```python
from build123d import *

# Parameters (mm, degrees)
BOSS_EXTRUDE1_DEPTH = 5


with BuildPart() as part:
    # Sketch1 → Boss-Extrude1 (new body)
    with BuildSketch(Plane(origin=(0, 0, 0), x_dir=(1, 0, 0), z_dir=(0, 1, 0))):
        with BuildLine():
            ThreePointArc((-40.530858986, 10), (-2.570543478, 38.792166423), (35.38977203, 10))
            Line((35.38977203, 10), (21.844456522, 10))
            Line((21.844456522, 10), (21.844456522, 0))
            Line((21.844456522, 0), (-26.985543478, 0))
            Line((-26.985543478, 0), (-26.985543478, 10))
            Line((-26.985543478, 10), (-40.530858986, 10))
        make_face()
    extrude(amount=BOSS_EXTRUDE1_DEPTH)


solid = part.part
```
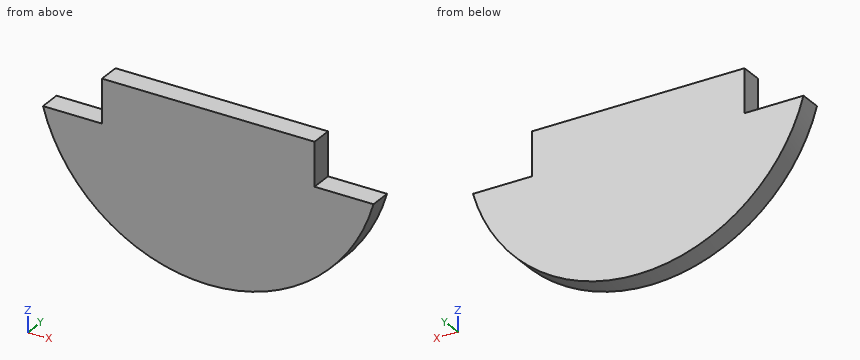
Check sheet for the modelled part. Datum: model origin and axes. Units: mm. Give positions to 0.01 mm unless a question says otherwise; leave off trailing zeros. Loops run counter-clockwise (first coordinate to the right, second up) from the corner with the lowest first, then second, coordinate; pieces in that order, holes last. Notation, with made-up numbers: (-21.5, -37) - (4.5, -37) arc R17 ccw to (4.5, -29) - close; hole circle Ø1 at (43.5, 44.5). An arc over 180 degrees is marked (long way). One line per question, with ' | ' between items. Start each with the question number.
1. Cross-section at C-C, the plane x = 26. Enter the section's corners in (y, z).
2. Gauge pin test, flat ends, axial feed: pin 1 Ø2 at (y, z) = (4.5, -26.5) entering from -X; pin 2 Ø1.5 at (y, z) = (1.5, -6) entering from -X. Record the tip position at first contact, or that the pin passes through.
3. Cross-section at B-B, the plane z = -5.5. Enter the section's corners in (x, y), plus the area to 3 significant figures.
4. Material ranges on line 1 along X through (y, z) = (2.1, -5.5); line 2 along X through (y, z) = (2.9, -17); line 3 along Z through (x, y) = (-30.5, 3), recorded low to high. Write a range as [from, to].
5. Cross-section at A-A, the plane y = 1.25. Enter the section's corners in (x, z).
Check result:
1) outline: (0, -26.53) - (5, -26.53) - (5, -10) - (0, -10) - close
2) pin 1: stops at x = -32.09 | pin 2: stops at x = -26.99
3) outline: (-26.99, 0) - (21.84, 0) - (21.84, 5) - (-26.99, 5) - close | area: 244 mm2
4) line 1: x = [-26.99, 21.84] | line 2: x = [-37.83, 32.69] | line 3: z = [-27.19, -10]
5) outline: (-40.53, -10) arc R39.42 ccw to (35.39, -10) - (21.84, -10) - (21.84, 0) - (-26.99, 0) - (-26.99, -10) - close
